```python
from build123d import *

# Parameters (mm, degrees)
SKETCH2_W           = 92
SKETCH2_H           = 87
BOSS_EXTRUDE1_DEPTH = 50
SKETCH4_W           = 50
SKETCH4_H           = 116
CUT_EXTRUDE1_DEPTH  = 27
SKETCH5_W           = 32
SKETCH5_H           = 50
BOSS_EXTRUDE2_DEPTH = 22
FILLET1_R           = 12
FILLET2_R           = 3
SKETCH7_R           = 6.5
CUT_EXTRUDE2_DEPTH  = 70
CHAMFER2_SIZE       = 3.5
CUT_EXTRUDE3_DEPTH  = 57
SKETCH10_R          = 9
CUT_EXTRUDE4_DEPTH  = 10


with BuildPart() as part:
    # Sketch2 → Boss-Extrude1 (new body)
    with BuildSketch(Plane.XY):
        Rectangle(SKETCH2_W, SKETCH2_H)
    extrude(amount=BOSS_EXTRUDE1_DEPTH)

    # Sketch4 → Cut-Extrude1 (cut)
    with BuildSketch(Plane.XY.offset(50)):
        with Locations((0, 43.5)):
            Rectangle(SKETCH4_W, SKETCH4_H)
    extrude(amount=-CUT_EXTRUDE1_DEPTH, mode=Mode.SUBTRACT)

    # Sketch5 → Boss-Extrude2 (add)
    with BuildSketch(Plane.XZ.offset(43.5)):
        with Locations((62, 25)):
            Rectangle(SKETCH5_W, SKETCH5_H)
        with Locations((-62, 25)):
            Rectangle(SKETCH5_W, SKETCH5_H)
    extrude(amount=-BOSS_EXTRUDE2_DEPTH)

    # Fillet1
    fillet1_edges = [part.edges().sort_by_distance(p)[0] for p in [
        (78, -32.5, 0),
        (78, -32.5, 50),
        (-78, -32.5, 50),
        (-78, -32.5, 0),
    ]]
    fillet(fillet1_edges, radius=FILLET1_R)

    # Fillet2
    fillet2_edges = [part.edges().sort_by_distance(p)[0] for p in [
        (-46, 11, 50),
        (-35.5, 43.5, 50),
        (25, 14.5, 50),
        (-25, 14.5, 50),
        (0, 43.5, 23),
        (25, 14.5, 23),
        (0, -14.5, 50),
        (-25, 43.5, 36.5),
        (-25, 14.5, 23),
        (0, -14.5, 23),
        (25, 43.5, 36.5),
        (46, 11, 0),
        (46, 11, 50),
        (56, -21.5, 0),
        (46, -21.5, 25),
        (56, -21.5, 50),
        (-46, 11, 0),
        (0, 43.5, 0),
        (-56, -21.5, 50),
        (0, -43.5, 50),
        (0, -43.5, 0),
        (78, -43.5, 25),
        (-78, -43.5, 25),
        (74.485281374, -43.5, 46.485281374),
        (74.485281374, -43.5, 3.514718626),
        (-74.485281374, -43.5, 3.514718626),
        (-74.485281374, -43.5, 46.485281374),
        (-78, -21.5, 25),
        (-56, -21.5, 0),
        (-74.485281374, -21.5, 3.514718626),
        (-74.485281374, -21.5, 46.485281374),
        (78, -21.5, 25),
        (74.485281374, -21.5, 46.485281374),
        (74.485281374, -21.5, 3.514718626),
        (-46, 43.5, 25),
        (46, 43.5, 25),
        (35.5, 43.5, 50),
    ]]
    fillet(fillet2_edges, radius=FILLET2_R)

    # Sketch7 → Cut-Extrude2 (cut)
    with BuildSketch(Plane.XY.offset(23)):
        with Locations((0, 28.5)):
            Circle(SKETCH7_R)
        with Locations((0, 1.5)):
            Circle(SKETCH7_R)
    extrude(amount=-CUT_EXTRUDE2_DEPTH, mode=Mode.SUBTRACT)

    # Chamfer2
    chamfer2_edges = [part.edges().sort_by_distance(p)[0] for p in [
        (-6.5, 28.5, 23),
        (-6.5, 1.5, 23),
    ]]
    chamfer(chamfer2_edges, length=CHAMFER2_SIZE)

    # Sketch9 → Cut-Extrude3 (cut)
    with BuildSketch(Plane(origin=(0, -21.5, 0), x_dir=(1, 0, 0), z_dir=(0, 1, 0))):
        with BuildLine():
            ThreePointArc((-62, -19.5), (-68.5, -26), (-62, -32.5))
            Line((-62, -32.5), (-62, -19.5))
        make_face()
        with BuildLine():
            Line((-62, -19.5), (-62, -32.5))
            ThreePointArc((-62, -32.5), (-57.403805922, -30.596194078), (-55.5, -26))
            ThreePointArc((-55.5, -26), (-57.403805922, -21.403805922), (-62, -19.5))
        make_face()
        with BuildLine():
            ThreePointArc((62, -19.5), (55.5, -26), (62, -32.5))
            Line((62, -32.5), (62, -19.5))
        make_face()
        with BuildLine():
            Line((62, -19.5), (62, -32.5))
            ThreePointArc((62, -32.5), (66.596194078, -30.596194078), (68.5, -26))
            ThreePointArc((68.5, -26), (66.596194078, -21.403805922), (62, -19.5))
        make_face()
    extrude(amount=-CUT_EXTRUDE3_DEPTH, mode=Mode.SUBTRACT)

    # Sketch10 → Cut-Extrude4 (cut)
    with BuildSketch(Plane(origin=(0, -21.5, 0), x_dir=(1, 0, 0), z_dir=(0, 1, 0))):
        with Locations(Location((-62, -26, 0), (0, 0, 270))):
            Circle(SKETCH10_R)
        with Locations(Location((62, -26, 0), (0, 0, 270))):
            Circle(SKETCH10_R)
    extrude(amount=-CUT_EXTRUDE4_DEPTH, mode=Mode.SUBTRACT)


solid = part.part
```
Part model, mm, in its own coordinate system. A direction names the side the tool comes from. Round coordinates to 2 decimals unless told otherwise and drop trailing zeros. Order: outer loops, then holes, each group sorted by start corner. A loop starts at its lowest first (then second) coordinate and runs counter-clockwise, first axis right, second up. Notation, with made-up numbers: M 73,-32 L 94,-32 A20 cw 94,-13 Z; hole C 31,38.25 d9. An arc over 180 degrees is marked long. Answer in a Markdown table with one row per item. Add a question column.
Q1. Mould opens along Y. For faces 6 (the face through (-1, -43.5, 25)), 7 (the face through (-0.846, 34.945, 9.886)), 8 (the face through (0.35, -13.6, 23.86)), 9 (the face through (-4.952, 33.041, 19.719)) say: +Y half, -Y half, draft (parallel to the pull), parting line (faces both ways), or undercut.
Q2. Pin check, flat tips, straight feed: pin 1 (3 mm diameter, centred on y = 7, z = 13.5, fed in from -X); pin 2 (1 mm diameter, centred on x = 45.5, y = -8, fed in from +Z); pin 3 (8.5 mm diameter, centred on x = -66.5, z = 28, fed in from +Y). Stop position of each tip, or through.
Q3. Cut at D-D on y = 28.5. Give the cut face in (x, z), and give its area (3 significant figures).
Q4. 3-axis set-ups, long thin cutter, end or side, ignore diameter. For faces 1 (the face through (46, 11, 25)), 2 (the face through (-68, -31.5, 29)), 3 (the face through (0.31, 42.64, 22.1)), 4 (the face through (-54, -21.5, 20)), 5 (the face through (-45.1, 8.45, 0.86)): which of +Z, -Z, +X, -X, +Y, -Y reach the whole face in a straight line?
Q5. Cut at C-C on x = 0. Give the cut face in (y, z), and give its area (3 significant figures).
Q6. Cut at B-B on y = -33.5. Give the cut face in (x, z).
Q7. Cut at A-A on z = 15.5. Give the cut face in (x, y), and give its area (3 significant figures).
Q8. Wall check: L1, parallel to X at y = -25, z = 26; L2, parallel to Y at x = 0, z = 12; L3, parallel to X at y = 24, z = 39. Give the ranges that are in metal, low to high. Write a range as from..to.
Established:
| question | item | result |
|---|---|---|
| 1 | face 6 | -Y half |
| 1 | face 7 | undercut |
| 1 | face 8 | +Y half |
| 1 | face 9 | undercut |
| 2 | pin 1 | stops at x = -46 |
| 2 | pin 2 | stops at z = 49.24 |
| 2 | pin 3 | stops at y = -21.5 |
| 3 | outline | M -46,3 A3 ccw -43,0 L -6.5,0 L -6.5,19.5 L -10,23 L -22,23 A3 cw -25,26 L -25,47 A3 ccw -28,50 L -43,50 A3 ccw -46,47 Z; M 6.5,0 L 43,0 A3 ccw 46,3 L 46,47 A3 ccw 43,50 L 28,50 A3 ccw 25,47 L 25,26 A3 cw 22,23 L 10,23 L 6.5,19.5 Z |
| 3 | area | 2,930 mm2 |
| 4 | face 1 | +Z, -Z, +X, +Y |
| 4 | face 2 | +Y |
| 4 | face 3 | +Z, +Y |
| 4 | face 4 | +Z, -Z, -X, +Y |
| 4 | face 5 | -Z, -X, +Y |
| 5 | outline | M -43.5,3 A3 ccw -40.5,0 L -5,0 L -5,19.5 L -8.5,23 L -11.5,23 A3 cw -14.5,26 L -14.5,47 A3 ccw -17.5,50 L -40.5,50 A3 ccw -43.5,47 Z; M 8,0 L 22,0 L 22,19.5 L 18.5,23 L 11.5,23 L 8,19.5 Z; M 35,0 L 40.5,0 A3 ccw 43.5,3 L 43.5,20 A3 ccw 40.5,23 L 38.5,23 L 35,19.5 Z |
| 5 | area | 2,150 mm2 |
| 6 | outline | M -78,12 A12 ccw -66,0 L 66,0 A12 ccw 78,12 L 78,38 A12 ccw 66,50 L -66,50 A12 ccw -78,38 Z; hole C -62,26 d13; hole C 62,26 d13 |
| 7 | outline | M -78,-40.5 A3 ccw -75,-43.5 L 75,-43.5 A3 ccw 78,-40.5 L 78,-24.5 A3 ccw 75,-21.5 L 49,-21.5 A3 cw 46,-18.5 L 46,40.5 A3 ccw 43,43.5 L -43,43.5 A3 ccw -46,40.5 L -46,-21.5 L -75,-21.5 A3 ccw -78,-24.5 Z; hole C 0,1.5 d13; hole C 0,28.5 d13 |
| 7 | area | 9,140 mm2 |
| 8 | L1 | x = -78..-71, -53..53, 71..78 |
| 8 | L2 | y = -43.5..-5, 8..22, 35..43.5 |
| 8 | L3 | x = -46..-25, 25..46 |
